Print and shaded views of the part. All mm, measured from the part's lowest x, y and z. Round coordinates to 2 decimals unless told otherwise and drop trailing zeros. Loops run counter-clockwise (first coordinate to the right, second up) from the corner with the lowest first, then second, coordinate; pieces in that order, holes last. Notation, with made-up numbers: (15.5, 19) -> (27.5, 19) arc R32 cw to (27.5, 53) -> close; hole circle Ø3 at (-21, 18). An arc over 180 degrees is marked (long way). Use a Markdown table: item, result.
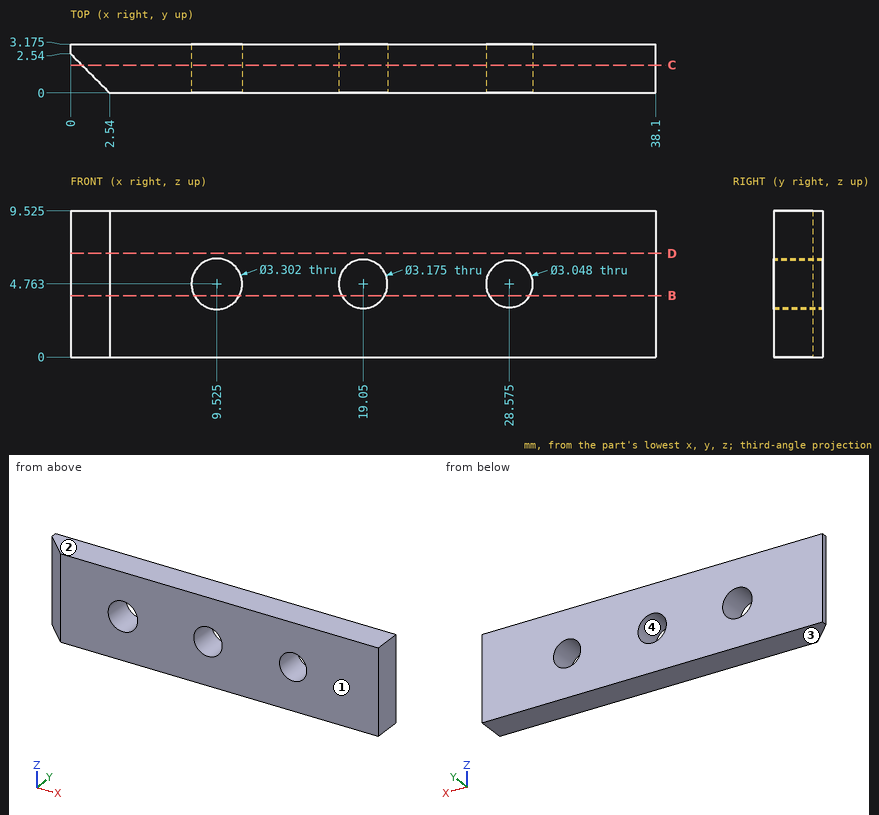
Q1. Drill centre lines: L1, parallel to Z at x = 28.5, y = 0.4 (1 decimal); L2, parallel to X at y = 0.8, z = 4.5 (1 decimal); L3, parallel to X at y = 2.15, z = 4.5 (1 decimal). Where is each one in solid material? Low to high. Write a range as from..to.
Results list:
| item | result |
|---|---|
| L1 | z = 0..3.2, 6.3..9.5 |
| L2 | x = 1.7..7.9, 11.2..17.5, 20.6..27.1, 30.1..38.1 |
| L3 | x = 0.4..7.9, 11.2..17.5, 20.6..27.1, 30.1..38.1 |
Q2. Band-saw the part on D-D, the plane z = 6.75. Give the cut face in (x, y) (1 decimal), plus the area to 3 significant figures.
Results list:
| item | result |
|---|---|
| outline | (0, 2.5) -> (2.5, 0) -> (38.1, 0) -> (38.1, 3.2) -> (0, 3.2) -> close |
| area | 118 mm² |
Q3. Band-saw the part on B-B, the plane z = 4. Give the cut face in (x, y) (1 decimal).
Results list:
| item | result |
|---|---|
| outline | (0, 2.5) -> (2.5, 0) -> (8.1, 0) -> (8.1, 3.2) -> (0, 3.2) -> close; (11, 0) -> (17.7, 0) -> (17.7, 3.2) -> (11, 3.2) -> close; (20.4, 0) -> (27.3, 0) -> (27.3, 3.2) -> (20.4, 3.2) -> close; (29.9, 0) -> (38.1, 0) -> (38.1, 3.2) -> (29.9, 3.2) -> close |
Q4. Band-saw the part on C-C, the plane y = 1.8. Give the number of separate pieces and of enclosed holes in the cut face, plus the area to 3 significant figures.
Results list:
| item | result |
|---|---|
| separate pieces | 1 |
| enclosed holes | 3 |
| area | 332 mm² |
Q5. Pull direction Z, two halves, no side cores. Call the marked faces 1, 2, 3 and 4: released by +Z, released by -Z, zero draft, split by the parting line, or undercut.
Results list:
| item | result |
|---|---|
| face 1 | zero draft |
| face 2 | released by +Z |
| face 3 | released by -Z |
| face 4 | undercut |
